Here's how the part is built. I have some questions about the finished solid (model axes, mm). A direction names the side the tool comes from. Coordinates: 2 decimals unless noted, no trailing zeros. Write each loop counter-clockwise with the first axis right and the second up, starting at its lowest first coordinate (ties: lowest second). Pieces come first, ordered by that corner, then holes. Notation, with made-up numbers: (56, 37) - (103, 37) arc R27 ccw to (103, 66) - close; hole circle Ø2 at (34, -16.75). An arc over 180 degrees is marked (long way). Answer in a Markdown table with one row per item. Add a question column.
Item 1: Imagine slicing it at C-C (x = 0.25). State how many separate pieces and enclosed holes the cut face has, plus the area to 3 significant figures.
Item 2: I'm going to push flat-ended pins straight in: pin 1 (3 mm diameter, centred on x = 7, y = -0.5, fed in from -Z); pin 2 (5 mm diameter, centred on x = 1, y = 2, fed in from -Z); pin 3 (0.8 mm diameter, centred on x = -2, z = 1.5, fed in from +Y); pin 4 (1.5 mm diameter, centred on x = 8.5, z = 3.5, fed in from -Y). Where does each tip first touch, or does it pass through?
Item 3: Imagine slicing it at A-A (y = 0). Please give me the cut outline in (x, z), plus the area to 3 significant figures.
Item 4: We'd pull the mould along Y, two halves only. Please class faces 1 (the face through (-0.1, 4.5, 4.4)), 2 (the face through (0.672, -10.004, 2.127)), 3 (the face through (12.83, 4.04, 3.11)), 4 (the face through (-0.2, 3.1, 6.3)): +Y half, -Y half, draft (parallel to the pull), parting line (faces both ways), or undercut.
Item 5: Which directions (+Z, -Z, +X, -X, +Y, -Y) give clear straight access to the entire face, cutting with the end or side of a thin tool? Please do faces 5 (the face through (-0.16, 7.71, 2.13)), 6 (the face through (0.141, -4.455, 4.483)).
Item 6: If I drill on probe 1 along Y at (x, z) = (0, 1.95); probe 2 along Y at (x, z) = (1.75, 6); probe 3 along X at (y, z) = (8.95, 2), over which ranges is the centre line in solid material (lowest first)? Write a range as from..to.
Item 7: Imagine slicing it at B-B (z = 1.25). Please give me the cut outline in (x, y).
from build123d import *

# Parameters (mm, degrees)
F0_R          = 13.45
F1_DEPTH      = 6.3
F3_DEPTH      = 10.1
F3_DEPTH_BACK = 10.1
F4_R          = 1.25
F5_DEPTH      = 10
F6_R          = 0.5
F7_SIZE       = 2.5


with BuildPart() as f1:
    # F0 (on Top) → F1 (new body)
    with BuildSketch(Plane.XY):
        Circle(F0_R)
    extrude(amount=F1_DEPTH)

    # F2 (on Right) → F3 (cut, two sides)
    with BuildSketch(Plane.YZ) as f3_sk:
        with BuildLine():
            Line((5.1, 0), (5.1, 2))
            ThreePointArc((5.1, 2), (0, 7.1), (-5.1, 2))
            Line((-5.1, 2), (-5.1, 0))
            Line((-5.1, 0), (5.1, 0))
        make_face()
    extrude(amount=F3_DEPTH, mode=Mode.SUBTRACT)
    extrude(f3_sk.sketch, amount=-F3_DEPTH_BACK, mode=Mode.SUBTRACT)

    # F4 (on face) → F5 (cut)
    with BuildSketch(Plane(origin=(0, 0, 0), x_dir=(1, 0, 0), z_dir=(0, 0, -1))):
        with Locations((0, 8.95)):
            Circle(F4_R)
        with Locations((0, -8.95)):
            Circle(F4_R)
    extrude(amount=-F5_DEPTH, mode=Mode.SUBTRACT)

    # F6
    f6_edges = [f1.edges().sort_by_distance(p)[0] for p in [
        (-13.45, 0, 0),
        (-1.25, -8.95, 0),
        (0, -5.1, 0),
        (-10.1, 0, 0),
        (10.1, 0, 0),
        (0, 5.1, 0),
        (-1.25, 8.95, 0),
        (-13.45, 0, 6.3),
    ]]
    fillet(f6_edges, radius=F6_R)

    # F7
    f7_edges = [f1.edges().sort_by_distance(p)[0] for p in [
        (-1.25, -8.95, 6.3),
        (-1.25, 8.95, 6.3),
    ]]
    chamfer(f7_edges, length=F7_SIZE)


solid = f1.part
Here are the results:
| question | item | result |
|---|---|---|
| 1 | separate pieces | 4 |
| 1 | enclosed holes | 0 |
| 1 | area | 67.1 mm2 |
| 2 | pin 1 | passes through |
| 2 | pin 2 | stops at z = 4.4 |
| 2 | pin 3 | stops at y = 13.35 |
| 2 | pin 4 | stops at y = -10.99 |
| 3 | outline | (-13.45, 0.5) arc R0.5 ccw to (-12.95, 0) - (-10.6, 0) arc R0.5 ccw to (-10.1, 0.5) - (-10.1, 6.3) - (-12.95, 6.3) arc R0.5 ccw to (-13.45, 5.8) - close; (10.1, 0.5) arc R0.5 ccw to (10.6, 0) - (12.95, 0) arc R0.5 ccw to (13.45, 0.5) - (13.45, 5.8) arc R0.5 ccw to (12.95, 6.3) - (10.1, 6.3) - close |
| 3 | area | 41.9 mm2 |
| 4 | face 1 | undercut |
| 4 | face 2 | undercut |
| 4 | face 3 | parting line |
| 4 | face 4 | draft |
| 5 | face 5 | +Z, -Z |
| 5 | face 6 | -Z |
| 6 | probe 1 | y = -13.45..-10.2, -7.7..-5.1, 5.1..7.7, 10.2..13.45 |
| 6 | probe 2 | y = -13.29..-11.92, -5.98..-3.16, 3.16..5.98, 11.92..13.29 |
| 6 | probe 3 | x = -10.04..-1.25, 1.25..10.04 |
| 7 | outline | circle Ø26.9 at (0, 0); hole (-10.1, -5.1) - (10.1, -5.1) - (10.1, 5.1) - (-10.1, 5.1) - close; hole circle Ø2.5 at (0, -8.95); hole circle Ø2.5 at (0, 8.95) |
